Here's how the part is built. I have some questions about the finished solid (model axes, mm). A direction names the side the tool comes from. Give positions to 0.01 mm unless a question says otherwise; leave off trailing zeros. Loops run counter-clockwise (first coordinate to the right, second up) from the corner with the lowest first, then second, coordinate; pieces in that order, holes last. Notation, with made-up numbers: (-0.75, 67) - (36.25, 67) arc R26 cw to (36.25, 106) - close; hole circle Ø7 at (58, -32.5). An arc over 180 degrees is marked (long way). Return JSON: item names as keys, results as strings. Group by question number.
(1) If we section it at B-B (z = 10): Please give me the cut outline in (x, y), then the cut area to 3 significant figures.
(2) If we mould it in two halves opening along Y, with no side actions, what happens to faces 3 (the flat face through (-24.608, -5, 10)), 4 (the flat face through (-46.608, -109, 10)), 5 (the flat face through (-28, -210.5, 10)), 6 (the flat face through (-39, 0, 10))? For each: released by +Y, released by -Y, zero draft, split by the parting line, or undercut.
(3) On a 3-axis mill with a long thin cutter (end or side, diameter ignored), from which of +Z, -Z, +X, -X, +Y, -Y can I reach the whole of each face in a straight line? I mean faces 1 (the flat face through (-28, -10, 10)), 2 (the cylindrical face through (-35.205, -4.93, 9.864)). Say none if no direction works.
(4) I need wall thicknesses on probe 1 along X at (y, z) = (-215.75, 10); probe 2 along Y at (x, z) = (-35.5, 4.5); probe 3 along X at (y, z) = (-56, 8). Which ranges of each line are inside material? Lowest first, please. Write a range as [from, to].
(5) If we section it at C-C (y = -27): Please give me the cut outline in (x, z), then the cut area to 3 significant figures.
(6) If we section it at D-D (x = -40): Please give me the cut outline in (y, z).
(7) For P1, Ø6, axis at y = -65.5, z = 13.5, coming from the +X side, with a flat end and sliding along its axis, tell me the tip position at first contact or that it passes through.
(8) If we section it at A-A (x = -27): Please give me the cut outline in (y, z), then the cut area to 3 significant figures.
Autodesk Inventor part; units mm, degrees
ref_plane "YZ Plane" through (0, 0, 0) normal (1, 0, 0) x (0, 1, 0)
ref_plane "XZ Plane" through (0, 0, 0) normal (0, 1, 0) x (-1, 0, 0)
ref_plane "XY Plane" through (0, 0, 0) normal (0, 0, 1) x (1, 0, 0)
ref_plane "Work Plane1" through (0, 0, 0) normal (0, 0, 1) x (1, 0, 0)
sketch "Sketch1" plane through (0, 0, 0) normal (0, 0, 1) x (1, 0, 0)
  line L0 (0, 0) -> (-19.6084, 0)
  line L1 (0, -10) -> (-19.6084, -10)
  line L2 (0, 0) -> (0, -10)
  line L3 (0, -210.5) -> (-19.6084, -210.5)
  line L4 (0, -220.5) -> (-19.6084, -220.5)
  line L5 (0, -220.5) -> (0, -210.5)
  line L6 (-52.6084, 0) -> (-46.6084, 0)
  line L7 (-46.6084, 0) -> (-46.6084, -220.5)
  line L8 (-46.6084, -220.5) -> (-52.6084, -220.5)
  line L9 (-52.6084, -220.5) -> (-52.6084, 0)
  line L10 (-35.1084, -220.5) -> (-35.1084, 29.5) construction
  line L11 (-29.1084, -220.5) -> (-29.1084, 29.5) construction
  line L12 (-46.6084, 0) -> (-24.6084, 0)
  line L13 (-24.6084, 0) -> (-24.6084, -10)
  line L14 (-24.6084, -10) -> (-46.6084, -10)
  line L15 (-46.6084, -10) -> (-46.6084, 0)
  line L16 (-46.6084, -220.5) -> (-24.6084, -220.5)
  line L17 (-24.6084, -220.5) -> (-24.6084, -210.5)
  line L18 (-24.6084, -210.5) -> (-46.6084, -210.5)
  line L19 (-46.6084, -210.5) -> (-46.6084, -220.5)
  line L20 (-19.6084, -10) -> (-19.6084, 0)
  line L21 (-19.6084, -220.5) -> (-19.6084, -210.5)
  dimension "d0" = 6
  dimension "d1" = 22
  dimension "d2" = 10
  dimension "d3" = 22
  dimension "d4" = 10
extrude "Extrusion1" add sketch "Sketch1" along normal blind 20 contours L6 L7 L8 L9 | L12 L13 L14 L7 | L7 L18 L17 L16
sketch "Sketch2" plane through (-52.6084, 0, 0) normal (0, 1, 0) x (1, 0, 0)
  circle A0 centre (20.5, 120.1) radius 3
  line L0 (0, 0) -> (28, 0)
  line L1 (0, 0) -> (0, -20)
  line L2 (28, -20) -> (0, -20)
  line L3 (28, 0) -> (28, -20)
  circle A1 centre (20.5, -10) radius 3.1
  point P0 (52.6084, 0)
  dimension "d7" = 6.2
  dimension "d8" = 10
extrude "Extrusion2" cut sketch "Sketch2" against normal through all contours A1
chamfer "Chamfer1" distance 10 angle 45 2 edges at (-46.6084, -10, 10) (-46.6084, -210.5, 10)
ref_plane "Work Plane2" through (0, 0, 10) normal (0, 0, 1) x (1, 0, 0)
properties part number "06_OPENTRONS_Microscope_Extraslide"
Values:
{
 "1": {"outline": "(-52.61, -220.5) - (-35.21, -220.5) - (-35.21, -210.5) - (-36.61, -210.5) - (-46.61, -200.5) - (-46.61, -20) - (-36.61, -10) - (-35.21, -10) - (-35.21, 0) - (-52.61, 0) - close; (-29.01, -220.5) - (-24.61, -220.5) - (-24.61, -210.5) - (-29.01, -210.5) - close; (-29.01, -10) - (-24.61, -10) - (-24.61, 0) - (-29.01, 0) - close", "area": "1,740 mm2"},
 "2": {"face 3": "zero draft", "face 4": "undercut", "face 5": "undercut", "face 6": "released by +Y"},
 "3": {"face 1": "+Z, -Z, +X", "face 2": "+Y, -Y"},
 "4": {"probe 1": "[-52.61, -35.21], [-29.01, -24.61]", "probe 2": "[-220.5, -210.5], [-10, 0]", "probe 3": "[-52.61, -46.61]"},
 "5": {"outline": "(-52.61, 0) - (-46.61, 0) - (-46.61, 20) - (-52.61, 20) - close", "area": "120 mm2"},
 "6": {"outline": "(-220.5, 0) - (-207.11, 0) - (-207.11, 20) - (-220.5, 20) - close; (-13.39, 0) - (0, 0) - (0, 20) - (-13.39, 20) - close"},
 "7": {"P1": "x = -46.61"},
 "8": {"outline": "(-220.5, 0) - (-210.5, 0) - (-210.5, 20) - (-220.5, 20) - close; (-10, 0) - (0, 0) - (0, 20) - (-10, 20) - close", "area": "400 mm2"}
}
